Here's how the part is built. I have some questions about the finished solid (model axes, mm). Face numbers are marked on the shaded views. A direction names the side the tool comes from. Round coordinates to 2 decimals unless told otherwise and drop trailing zeros. Order: outer loops, then holes, each group sorted by start corner. A loop starts at its lowest first (then second) coordinate and runs counter-clockwise, first axis right, second up. Notation, with made-up numbers: M -4.5,60 L 35.5,60 A17 ccw 35.5,83 Z; hole C 13,70.5 d2. An arc over 180 degrees is marked long. Answer as CSV lines item,"result". Start each with the question number.
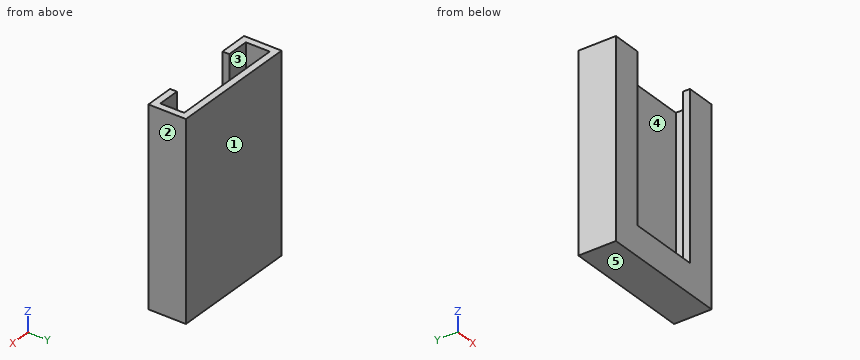
```python
from build123d import *

# Parameters (mm, degrees)
F0_W     = 96.52
F0_H     = 144.78
F1_DEPTH = 27.94
F2_T     = -5.08
F3_W     = 52.832
F3_H     = 122.936
F4_DEPTH = 7.62


with BuildPart() as f1:
    # F0 (on Front) → F1 (new body)
    with BuildSketch(Plane.XZ):
        with Locations((-12.624722, -18.957326)):
            Rectangle(F0_W, F0_H)
    extrude(amount=F1_DEPTH)

    # F2
    f2_openings = [f1.faces().sort_by_distance(p)[0] for p in [
        (-12.624722, -13.97, 53.432674),
    ]]
    offset(amount=F2_T, openings=f2_openings)

    # F3 (on face) → F4 (cut)
    with BuildSketch(Plane.XZ.offset(27.94)):
        with Locations((-12.624722, -8.035326)):
            Rectangle(F3_W, F3_H)
    extrude(amount=-F4_DEPTH, mode=Mode.SUBTRACT)


solid = f1.part
```
Item 1: If we section it at C-C on y = -11.5: Please give me the cut outline in (x, z).
Item 2: Which directions (+Z, -Z, +X, -X, +Y, -Y) give clear straight access to the entire face, cutting with the end or side of a thin tool? Please do the marked faces 4 and 5.
Item 3: If we section it at A-A on z = -63.5: Please give me the cut outline in (x, y), and give its area (3 significant figures).
Item 4: We'd pull the mould along X, two halves only. Please class the marked faces 1, 2 and 3: pulls with the +X half, pulls with the -X half, needs draft (parallel to the pull), parting line crosses it, or undercut.
Item 5: If I drill on line 1 along X through (y, z) = (-25.75, -60); line 2 along X through (y, z) = (-7.5, -78); line 3 along Y through (x, z) = (30.5, -1), over which ranges is the centre line in solid material (lowest first)?
Item 6: If we section it at B-B on x = 28.5: Please give me the cut outline in (y, z).
Item 7: For P1, Ø8, axis at x = -13.5, y = -23, coming from the +Z side; P2, Ø5, axis at x = -24.5, y = -15.5, coming from the +Z side, each with a flat end and sliding along its axis, tell me the tip position at first contact or that it passes through.
Geometry says:
1,outline,"M -60.88,-91.35 L 35.64,-91.35 L 35.64,53.43 L 30.56,53.43 L 30.56,-86.27 L -55.8,-86.27 L -55.8,53.43 L -60.88,53.43 Z"
2,face 4,"+Z"
2,face 5,"-Z, +X, -X, +Y, -Y"
3,outline,"M -60.88,-27.94 L -39.04,-27.94 L -39.04,-22.86 L -55.8,-22.86 L -55.8,-5.08 L 30.56,-5.08 L 30.56,-22.86 L 13.79,-22.86 L 13.79,-27.94 L 35.64,-27.94 L 35.64,0 L -60.88,0 Z"
3,area,"893 mm²"
4,face 1,"needs draft"
4,face 2,"pulls with the +X half"
4,face 3,"undercut"
5,line 1,"-60.88 to -39.04, 13.79 to 35.64"
5,line 2,"-60.88 to -55.8, 30.56 to 35.64"
5,line 3,"-27.94 to -22.86, -5.08 to 0"
6,outline,"M -27.94,-91.35 L 0,-91.35 L 0,53.43 L -5.08,53.43 L -5.08,-86.27 L -22.86,-86.27 L -22.86,53.43 L -27.94,53.43 Z"
7,P1,"z = -69.5"
7,P2,"z = -86.27"
